Geometry check sheet. Reference: the model listing, model coordinates, mm. Face numbers are marked on the shaded views. A direction names the side the tool comes from. Give positions to 0.01 mm unless a question says otherwise; leave off trailing zeros. Loops run counter-clockwise (first coordinate to the right, second up) from the corner with the lowest first, then second, coordinate; pieces in that order, holes last. Notation, with made-up numbers: (11, -21.5) -> (34, -21.5) arc R12 cw to (34, -6.5) -> close; hole circle Ø6 at (63, 48.25). An arc over 180 degrees is marked (long way). Write item = value, one per line.
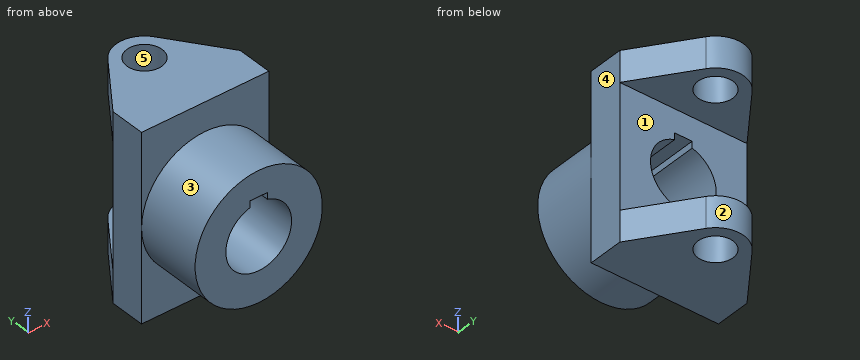
```python
from build123d import *

# Parameters (mm, degrees)
SKETCH1_R           = 29
BOSS_EXTRUDE1_DEPTH = 30
SKETCH3_W           = 58
SKETCH3_H           = 84
BOSS_EXTRUDE2_DEPTH = 16
SKETCH4_R           = 8
EXTRUDE_Q_DEPTH     = 14
CUT_EXTRUDE1_DEPTH  = 93.379651439


with BuildPart() as part:
    # Sketch1 → Boss-Extrude1 (new body)
    with BuildSketch(Plane(origin=(0, 0, 0), x_dir=(-1, 0, 0), z_dir=(0, 1, 0))):
        with Locations(Location((0, 0, 0), (0, 0, 90))):
            Circle(SKETCH1_R)
    extrude(amount=BOSS_EXTRUDE1_DEPTH)

    # Sketch3 → Boss-Extrude2 (add)
    with BuildSketch(Plane(origin=(0, 30, 0), x_dir=(-1, 0, 0), z_dir=(0, 1, 0))):
        Rectangle(SKETCH3_W, SKETCH3_H)
    extrude(amount=BOSS_EXTRUDE2_DEPTH)

    # Sketch4 → Extrude q (add)
    with BuildSketch(Plane.XY.offset(42)):
        with BuildLine():
            Line((-29, 30), (-29, 46))
            Line((-29, 46), (-10.54585016, 71.60164748))
            ThreePointArc((-10.54585016, 71.60164748), (0, 77), (10.54585016, 71.60164748))
            Line((10.54585016, 71.60164748), (29, 46))
            Line((29, 46), (29, 30))
            Line((29, 30), (-29, 30))
        make_face()
        with Locations((0, 64)):
            Circle(SKETCH4_R, mode=Mode.SUBTRACT)
    extrude_q = extrude(amount=-EXTRUDE_Q_DEPTH)

    # Mirror1: Extrude q across plane
    add(extrude_q.mirror(Plane.XY))

    # Sketch5 → Cut-Extrude1 (cut, through all)
    with BuildSketch(Plane.XZ):
        with BuildLine():
            Line((-4, 17.456832295), (4, 17.456832295))
            Line((4, 17.456832295), (4, 14.456832295))
            ThreePointArc((4, 14.456832295), (0, -15), (-4, 14.456832295))
            Line((-4, 14.456832295), (-4, 17.456832295))
        make_face()
    extrude(amount=-CUT_EXTRUDE1_DEPTH, mode=Mode.SUBTRACT)


solid = part.part
```
Item 1: Section check B-B, the plane x = 0. Record the cut outline in (y, z).
Answer:
outline = (0, -29) -> (30, -29) -> (30, -42) -> (56, -42) -> (56, -28) -> (46, -28) -> (46, -15) -> (0, -15) -> close; (0, 17.46) -> (46, 17.46) -> (46, 28) -> (56, 28) -> (56, 42) -> (30, 42) -> (30, 29) -> (0, 29) -> close; (72, -42) -> (77, -42) -> (77, -28) -> (72, -28) -> close; (72, 28) -> (77, 28) -> (77, 42) -> (72, 42) -> close
Item 2: Tool access check on the marked faces 1 and 2. Record the directions out of +Z, -Z, +X, -X, +Y, -Y that give a thin tool (end or side, any length) a straight path to the whole face; none if there is none.
Answer:
face_1 = +X, -X, +Y
face_2 = +Z, -Z, +Y
Item 3: Thickness scan on L1, parallel to Z at x = 5.5, y = 53; L2, parallel to Z at x = 0, y = 23; L3, parallel to X at y = 34.5, z = 0. Record the ranges inside material, lowest first. Write a range as [from, to].
Answer:
L1 = [-42, -28], [28, 42]
L2 = [-29, -15], [17.46, 29]
L3 = [-29, -15], [15, 29]
Item 4: Draft check along X on the marked faces 3, 4 and 5. Enter one of: +X half, -X half, draft (parallel to the pull), parting line (faces both ways), or undercut.
Answer:
face_3 = parting line
face_4 = +X half
face_5 = undercut
Item 5: Section check A-A, the plane z = -32. Record the cut outline in (x, y), plus the area to 3 significant figures.
Answer:
outline = (-29, 30) -> (29, 30) -> (29, 46) -> (10.55, 71.6) arc R13 ccw to (-10.55, 71.6) -> (-29, 46) -> close; hole circle Ø16 at (0, 64)
area = 1,820 mm^2
Item 6: Gauge pin test, flat ends, axial feed: pin 1 (2.5 mm diameter, centred on y = 24.5, z = 15, fed in from -X); pin 2 (5 mm diameter, centred on x = -5, y = 23, fed in from -Z); pin 3 (1.5 mm diameter, centred on y = 22.5, z = 16, fed in from +X); pin 4 (2 mm diameter, centred on x = -3, z = 24, fed in from -Y). Record the tip position at first contact, or that the pin passes through.
Answer:
pin_1 = -25.53
pin_2 = -28.89
pin_3 = 24.67
pin_4 = 0
Item 7: Section check C-C, the plane y = 38.5. Record the cut outline in (x, z), plus the area to 3 significant figures.
Answer:
outline = (-29, -42) -> (29, -42) -> (29, 42) -> (-29, 42) -> close; hole (-4, 14.46) arc R15 ccw (long way) to (4, 14.46) -> (4, 17.46) -> (-4, 17.46) -> close
area = 4,140 mm^2
Item 8: Section check D-D, the plane y = 54. Record the cut outline in (x, z).
Answer:
outline = (-23.23, -42) -> (23.23, -42) -> (23.23, -28) -> (-23.23, -28) -> close; (-23.23, 28) -> (23.23, 28) -> (23.23, 42) -> (-23.23, 42) -> close
